from build123d import *

# Parameters (mm, degrees)
F0_W     = 38.1
F0_H     = 31.75
F1_DEPTH = 25.4
F4_DEPTH = 25.4


# Not quite as in the source:
# - a feature of the source that left no trace in its solid (it failed there, or was rolled back) is left out


with BuildPart() as f1:
    # F0 (on Front) → F1 (new body)
    with BuildSketch(Plane.XZ):
        with Locations((-31.4665150195, 15.875)):
            Rectangle(F0_W, F0_H)
    extrude(amount=F1_DEPTH)

    # F2 (on face) → F4 (cut)
    with BuildSketch(Plane.YZ.offset(-12.4165150195)):
        Polygon((-25.4, 7.9906463393), (-4.3392399561, 31.75), (-25.4, 31.75), align=None)
    extrude(amount=-F4_DEPTH, mode=Mode.SUBTRACT)


solid = f1.part
Verification items for the finished model (mm, model axes). A direction names the side the tool comes from. Round coordinates to 2 decimals unless told otherwise and drop trailing zeros. Order: outer loops, then holes, each group sorted by start corner. A loop starts at its lowest first (then second) coordinate and runs counter-clockwise, first axis right, second up. Notation, with made-up numbers: (28.5, 14.25) -> (65.5, 14.25) arc R33 ccw to (65.5, 49.25) -> close; hole circle Ø5 at (-26, -37.5). An arc over 180 degrees is marked (long way). Put each result on its own line as item: value.
1) Material ranges on line 1 (X direction, y = -13.25, z = 22.5); line 2 (Y direction, x = -24.5, z = 8); line 3 (Z direction, x = -28, y = -8.5), recorded low to high.
Final values:
line 1: x = -50.52 to -37.82
line 2: y = -25.39 to 0
line 3: z = 0 to 27.06
2) Section check C-C (z = 22.5). Record the cut outline in (x, y), then the cut area to 3 significant figures.
Final values:
outline: (-50.52, -25.4) -> (-37.82, -25.4) -> (-37.82, -12.54) -> (-12.42, -12.54) -> (-12.42, 0) -> (-50.52, 0) -> close
area: 641 mm^2
3) Section check B-B (y = -9.75). Record the cut outline in (x, z), then the cut area to 3 significant figures.
Final values:
outline: (-50.52, 0) -> (-12.42, 0) -> (-12.42, 25.65) -> (-37.82, 25.65) -> (-37.82, 31.75) -> (-50.52, 31.75) -> close
area: 1,050 mm^2
4) Section check A-A (x = -16.5). Record the cut outline in (y, z), then the cut area to 3 significant figures.
Final values:
outline: (-25.4, 0) -> (0, 0) -> (0, 31.75) -> (-4.34, 31.75) -> (-25.4, 7.99) -> close
area: 556 mm^2
5) Set-up check for faces 1 (the flat face through (-24.94, -15.02, 19.7)), 2 (the flat face through (-12.417, -10, 12)): record each of +Z, -Z, +X, -X, +Y, -Y from which the full face is reachable in a straight line by a thin tool's end or side.
Final values:
face 1: +Z, +X, -Y
face 2: +Z, -Z, +X, +Y, -Y
